Here's how the part is built. I have some questions about the finished solid (model axes, mm). Face numbers are marked on the shaded views. A direction names the side the tool comes from. Coordinates: 2 decimals unless noted, no trailing zeros. Loops run counter-clockwise (first coordinate to the right, second up) from the corner with the lowest first, then second, coordinate; pieces in that order, holes last.
```python
from build123d import *

# Parameters (mm, degrees)
SKETCH1_R               = 21
SKETCH1_R_2             = 20
BOSS_EXTRUDE1_DEPTH     = 100
CUT_EXTRUDE1_REACH      = 112.476
CUT_EXTRUDE1_END_RADIUS = 20
SKETCH2_R               = 6.5
CUT_EXTRUDE3_REACH      = 112.476
SKETCH5_R               = 3
BOSS_EXTRUDE2_START     = 1
SKETCH3_R               = 21
BOSS_EXTRUDE2_DEPTH     = 1
CUT_EXTRUDE2_REACH      = 107.276
SKETCH4_R               = 6.5


with BuildPart() as part:
    # Sketch1 → Boss-Extrude1 (new body)
    with BuildSketch(Plane.XY):
        Circle(SKETCH1_R)
        Circle(SKETCH1_R_2, mode=Mode.SUBTRACT)
    extrude(amount=BOSS_EXTRUDE1_DEPTH)

    # Cut-Extrude1: up to this cylinder (the profile starts outside it)
    cut_extrude1_end = Plane(origin=(0, 0, 80), z_dir=(0, 0, -1)) * Cylinder(CUT_EXTRUDE1_END_RADIUS, 265.952, mode=Mode.PRIVATE)
    # Sketch2 → Cut-Extrude1 (cut, up to the surface)
    with BuildSketch(Plane.ZY.offset(21), mode=Mode.PRIVATE) as cut_extrude1_sk1:
        with Locations((80, 0)):
            Circle(SKETCH2_R)
    cut_extrude1_tool1 = extrude(cut_extrude1_sk1.sketch, amount=-CUT_EXTRUDE1_REACH, mode=Mode.PRIVATE) - cut_extrude1_end
    add(cut_extrude1_tool1.solids().sort_by_distance((-21, 0, 80))[0], mode=Mode.SUBTRACT)

    # Sketch5 → Cut-Extrude3 (cut, up to next)
    with BuildSketch(Plane.ZY.offset(21), mode=Mode.PRIVATE) as cut_extrude3_sk1:
        with Locations((80, 0)):
            Circle(SKETCH5_R)
    cut_extrude3_tool1 = extrude(cut_extrude3_sk1.sketch, amount=-CUT_EXTRUDE3_REACH, mode=Mode.PRIVATE) & part.part
    add(cut_extrude3_tool1.solids().sort_by_distance((-21, 0, 80))[0], mode=Mode.SUBTRACT)

    # Sketch3 → Boss-Extrude2 (add)
    with BuildSketch(Plane(origin=(0, 0, 0), x_dir=(-1, 0, 0), z_dir=(0, 0, -1)).offset(BOSS_EXTRUDE2_START)):
        Circle(SKETCH3_R)
    extrude(amount=-BOSS_EXTRUDE2_DEPTH)

    # Sketch4 → Cut-Extrude2 (cut, up to next)
    with BuildSketch(Plane(origin=(0, 0, -1), x_dir=(-1, 0, 0), z_dir=(0, 0, -1)), mode=Mode.PRIVATE) as cut_extrude2_sk1:
        with Locations((2.632276964, 6.486225249)):
            Circle(SKETCH4_R)
    cut_extrude2_tool1 = extrude(cut_extrude2_sk1.sketch, amount=-CUT_EXTRUDE2_REACH, mode=Mode.PRIVATE) & part.part
    add(cut_extrude2_tool1.solids().sort_by_distance((-2.632277, 6.486225, -1))[0], mode=Mode.SUBTRACT)


solid = part.part
```
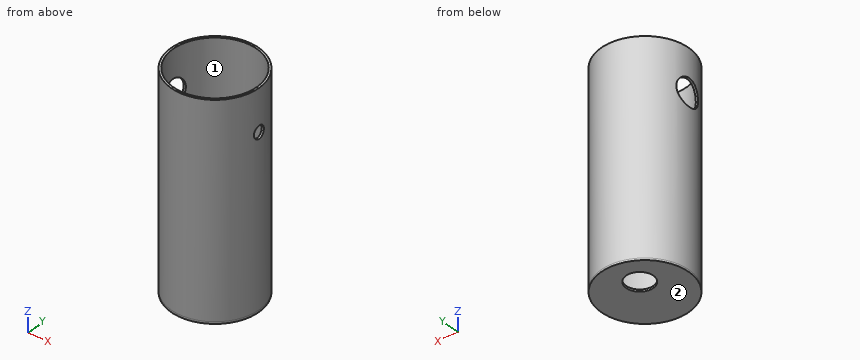
1. For pin 1 (4 mm diameter, centred on x = 6.5, y = -7.5, fed in from +Z); pin 2 (12 mm diameter, centred on x = -16.5, z = 25.5, fed in from +Y); pin 3 (11.5 mm diameter, centred on y = 0, z = 80, fed in from -X); pin 4 (11.5 mm diameter, centred on x = -2.63, y = 6.49, fed in from +Z), each with a flat end and sliding along its axis, tell me the tip position at first contact or that it passes through.
2. On a 3-axis mill with a long thin cutter (end or side, diameter ignored), from which of +Z, -Z, +X, -X, +Y, -Y can I reach the whole of each face in a straight line? I mean the marked faces 1 and 2. Say none if no direction works.
3. I want a section at C-C (z = 80). Please give me the cut outline in (x, y), then the cut area to 3 significant figures.
4. I want a section at D-D (x = 12). Please give me the cut outline in (y, z).
5. I want a section at A-A (x = 0.5). Please give me the cut outline in (y, z).
6. I want a section at B-B (y = -4.5). Please give me the cut outline in (x, z), then the cut area to 3 significant figures.
7. I need wall thicknesses on line 1 along Y through (x, z) = (0, 43.5); line 2 along X through (y, z) = (9.5, 7); line 3 along Z through (x, y) = (6, -5.5). Which ranges of each line are inside material? Lowest first, please.
Response values:
1. pin 1: stops at z = 0
1. pin 2: stops at y = 18.19
1. pin 3: stops at x = 19.16
1. pin 4: passes through
2. face 1: +Z
2. face 2: -Z, +X, -X, +Y, -Y
3. outline: (-19.97, -6.5) arc R21 ccw to (20.78, -3) - (19.77, -3) arc R20 cw to (-18.91, -6.5) - close; (-19.97, 6.5) - (-18.91, 6.5) arc R20 cw to (19.77, 3) - (20.78, 3) arc R21 ccw to start
3. area: 110 mm2
4. outline: (-17.23, -1) - (17.23, -1) - (17.23, 100) - (16, 100) - (16, 0) - (-16, 0) - (-16, 100) - (-17.23, 100) - close
5. outline: (-20.99, -1) - (0.79, -1) - (0.79, 0) - (-19.99, 0) - (-19.99, 100) - (-20.99, 100) - close; (12.18, -1) - (20.99, -1) - (20.99, 100) - (19.99, 100) - (19.99, 0) - (12.18, 0) - close
6. outline: (-20.51, -1) - (20.51, -1) - (20.51, 100) - (19.49, 100) - (19.49, 0) - (-19.49, 0) - (-19.49, 75.31) - (-20.51, 75.31) - close; (-20.51, 84.69) - (-19.49, 84.69) - (-19.49, 100) - (-20.51, 100) - close
6. area: 236 mm2
7. line 1: y = -21 to -20, 20 to 21
7. line 2: x = -18.73 to -17.6, 17.6 to 18.73
7. line 3: z = -1 to 0
